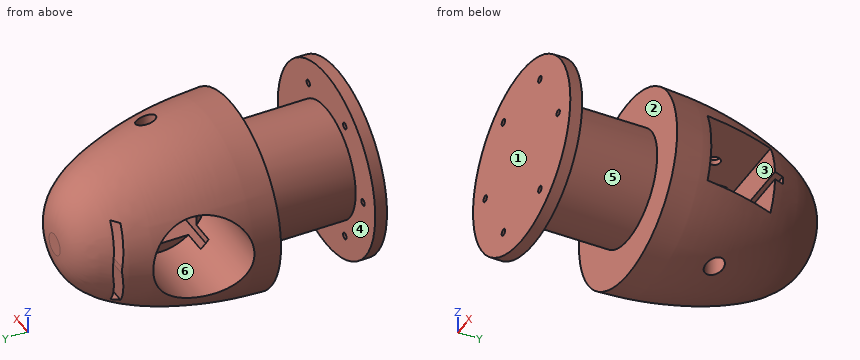
```python
from build123d import *

# Parameters (mm, degrees)
CUT_EXTRUDE1_DEPTH      = 52.443023194
CUT_EXTRUDE1_DEPTH_BACK = 12.7
SKETCH5_R               = 24.444582539
CUT_EXTRUDE2_DEPTH      = 66.04
SKETCH10_R              = 3.175
CUT_EXTRUDE3_DEPTH      = 52.443023194
CUT_EXTRUDE3_DEPTH_BACK = 52.443023194
SKETCH12_R              = 5.08
CUT_EXTRUDE4_DEPTH      = 43.688
CUT_EXTRUDE4_DEPTH_BACK = 0.508
SKETCH13_R              = 5.08
CUT_EXTRUDE5_DEPTH      = 43.688
SKETCH19_W              = 74.622524606
SKETCH19_H              = 50.8
SKETCH16_R              = 1.778
CUT_EXTRUDE6_DEPTH      = 7.62
CUT_EXTRUDE7_DEPTH      = 19.05


with BuildPart() as part:
    # Sketch3 → Revolve2 (revolve)
    with BuildSketch(Plane(origin=(0, 0, 0), x_dir=(0, 0, -1), z_dir=(1, 0, 0))):
        with BuildLine():
            Line((0, 0), (0, 152.4))
            Line((0, 152.4), (5.775087988, 152.4))
            add(Edge.make_bspline(
                [(5.775087988, 152.4), (26.104606075, 152.101942681), (56.331539835, 91.459760386), (51.027706874, 40.286381735), (50.8, 0)],
                knots=[0, 0, 0, 0, 0.330383286, 1, 1, 1, 1], degree=3))
            Line((50.8, 0), (0, 0))
        make_face()
    revolve(axis=Axis((0, 0, 0), (0, 1, 0)))

    # Sketch4 → Cut-Extrude1 (cut, two sides)
    with BuildSketch(Plane(origin=(0, 0, 0), x_dir=(0, 0, -1), z_dir=(1, 0, 0))) as cut_extrude1_sk:
        Polygon((-19.3675, 114.681), (-2.159, 114.681), (-2.159, 119.761), (2.159, 119.761), (2.159, 114.681), (19.3675, 114.681), (19.3675, 76.2), (-19.3675, 76.2), align=None)
    extrude(amount=CUT_EXTRUDE1_DEPTH, mode=Mode.SUBTRACT)
    extrude(cut_extrude1_sk.sketch, amount=-CUT_EXTRUDE1_DEPTH_BACK, mode=Mode.SUBTRACT)

    # Sketch5 → Cut-Extrude2 (cut)
    with BuildSketch(Plane(origin=(0, 0, 0), x_dir=(0, 0, -1), z_dir=(1, 0, 0))):
        with Locations((0, 95.4405)):
            Circle(SKETCH5_R)
    extrude(amount=-CUT_EXTRUDE2_DEPTH, mode=Mode.SUBTRACT)

    # Sketch10 → Cut-Extrude3 (cut, two sides)
    with BuildSketch(Plane.XY) as cut_extrude3_sk:
        with Locations((15.896399951, 95.3)):
            Circle(SKETCH10_R)
    extrude(amount=CUT_EXTRUDE3_DEPTH, mode=Mode.SUBTRACT)
    extrude(cut_extrude3_sk.sketch, amount=-CUT_EXTRUDE3_DEPTH_BACK, mode=Mode.SUBTRACT)

    # Sketch12 → Cut-Extrude4 (cut, two sides)
    with BuildSketch(Plane.XY.offset(22.86)) as cut_extrude4_sk:
        with Locations((15.896399951, 95.3)):
            Circle(SKETCH12_R)
    extrude(amount=CUT_EXTRUDE4_DEPTH, mode=Mode.SUBTRACT)
    extrude(cut_extrude4_sk.sketch, amount=-CUT_EXTRUDE4_DEPTH_BACK, mode=Mode.SUBTRACT)

    # Sketch13 → Cut-Extrude5 (cut)
    with BuildSketch(Plane.XY.offset(-22.86)):
        with Locations((15.896399951, 95.3)):
            Circle(SKETCH13_R)
    extrude(amount=-CUT_EXTRUDE5_DEPTH, mode=Mode.SUBTRACT)

    # Sketch19 → Cut-Revolve1 (revolve, cut)
    with BuildSketch(Plane.XY):
        with Locations((67.791262303, 31.75)):
            Rectangle(SKETCH19_W, SKETCH19_H)
    revolve(axis=Axis((0, 0, 0), (0, 1, 0)), mode=Mode.SUBTRACT)

    # Sketch16 → Cut-Extrude6 (cut)
    with BuildSketch(Plane.XZ):
        with Locations((38.1, 0)):
            Circle(SKETCH16_R)
        with Locations((19.05, -32.995567884)):
            Circle(SKETCH16_R)
        with Locations((-19.05, -32.995567884)):
            Circle(SKETCH16_R)
        with Locations((-38.1, 0)):
            Circle(SKETCH16_R)
        with Locations((-19.05, 32.995567884)):
            Circle(SKETCH16_R)
        with Locations((19.05, 32.995567884)):
            Circle(SKETCH16_R)
    extrude(amount=-CUT_EXTRUDE6_DEPTH, mode=Mode.SUBTRACT)

    # Sketch20 → Cut-Extrude7 (cut)
    with BuildSketch(Plane.ZY.offset(35.56)):
        Polygon((23.022216919, 130.648515898), (1.796344675, 133.35), (-1.796344675, 133.35), (-23.022216919, 130.648515898), (-23.681538514, 134.405336053), (-2.037826091, 137.16), (2.037826091, 137.16), (23.681538514, 134.405336053), align=None)
    extrude(amount=-CUT_EXTRUDE7_DEPTH, mode=Mode.SUBTRACT)


solid = part.part
```
Input: part model. Units: mm. Frame: model coordinates. Face numbers are marked on the shaded views. A direction names the side the tool comes from. Round coordinates to 2 decimals unless told otherwise and drop trailing zeros. Use one line per item in the form item = value. Start each with the question number.
Item 1: Material intervals for L1, parallel to Y at x = -21.5, z = -25; L2, parallel to Y at x = -33.5, z = 12.5; L3, parallel to Y at x = -15, z = 0, sorted ascending. Write a range as from..to.
Item 2: Contact query for flat-ended pins moving along their axis: pin 1 Ø4.5 at (x, z) = (-20.5, 0) entering from -Y; pin 2 Ø1.5 at (x, z) = (-32.5, -15) entering from +Y; pin 3 Ø7 at (y, z) = (133, 4.5) entering from -X; pin 4 Ø4.5 at (y, z) = (77.5, 17.5) entering from +X. Output: stop coordinate, or through.
Item 3: Section query A-A on x = -19.05. Count the separate pieces of the cut face and the enclosed holes in it, then the cut area to 3 significant figures.
Item 4: Mould query, pull axis Z, two halves, no side actions, for the marked faces 4, 5 and 6. Classes: pulls with the +Z half, pulls with the -Z half, needs draft (parallel to the pull), parting line crosses it, or undercut.
Item 5: Set-up query: the marked faces 1, 2 and 3. Return all of +Z, -Z, +X, -X, +Y, -Y with unobstructed straight access to the full face (end or side cutting, diameter ignored); none if empty.
Ans:
q1.L1 = 0..6.35, 57.15..134.41
q1.L2 = 0..6.35, 57.15..74.43, 116.45..129.34
q1.L3 = 0..71, 119.89..150.74
q2.pin_1 = 0
q2.pin_2 = 130.73
q2.pin_3 = -35.44
q2.pin_4 = 47.39
q3.separate_pieces = 3
q3.enclosed_holes = 2
q3.area = 7,800 mm^2
q4.face_4 = needs draft
q4.face_5 = parting line crosses it
q4.face_6 = undercut
q5.face_1 = +Z, -Z, +X, -X, -Y
q5.face_2 = none
q5.face_3 = +X
